from build123d import *

# Parameters (mm, degrees)
SKETCH1_W           = 50
SKETCH1_H           = 5
BOSS_EXTRUDE1_DEPTH = 50
SKETCH2_R           = 8
CUT_EXTRUDE1_DEPTH  = 50
SKETCH3_R           = 5
SKETCH3_R_2         = 4
BOSS_EXTRUDE2_DEPTH = 19
BOSS_EXTRUDE4_DEPTH = 19


with BuildPart() as part:
    # Sketch1 → Boss-Extrude1 (new body)
    with BuildSketch(Plane.XY):
        with Locations((25, -2.5)):
            Rectangle(SKETCH1_W, SKETCH1_H)
    extrude(amount=-BOSS_EXTRUDE1_DEPTH)

    # Sketch2 → Cut-Extrude1 (cut)
    with BuildSketch(Plane.XY):
        Circle(SKETCH2_R)
    extrude(amount=-CUT_EXTRUDE1_DEPTH, mode=Mode.SUBTRACT)



with BuildPart() as body_2:
    # Sketch3 → Boss-Extrude2 (new body)
    with BuildSketch(Plane(origin=(0, 0, -15.5), x_dir=(-1, 0, 0), z_dir=(0, 0, -1))):
        Circle(SKETCH3_R)
        Circle(SKETCH3_R_2, mode=Mode.SUBTRACT)
    extrude(amount=BOSS_EXTRUDE2_DEPTH)


with BuildPart() as part_1:
    add(part.part)

    add(body_2.part)  # Boss-Extrude4 merges body 2
    # Sketch8 → Boss-Extrude4 (add)
    with BuildSketch(Plane(origin=(0, 0, -34.5), x_dir=(-1, 0, 0), z_dir=(0, 0, -1))):
        with BuildLine():
            Line((-4, 0), (-10, 0))
            Line((-10, 0), (-10, -5))
            Line((-10, -5), (0, -5))
            Line((0, -5), (0, -4))
            ThreePointArc((0, -4), (-2.828427125, -2.828427125), (-4, 0))
        make_face()
    extrude(amount=-BOSS_EXTRUDE4_DEPTH)


solid = part_1.part
Work out the finished part from the listing and answer in its coordinate system (mm). A direction names the side the tool comes from. Round coordinates to 2 decimals unless told otherwise and drop trailing zeros. Loops run counter-clockwise (first coordinate to the right, second up) from the corner with the lowest first, then second, coordinate; pieces in that order, holes last. Notation, with made-up numbers: (55.5, 8) -> (77.5, 8) arc R27 cw to (77.5, 28) -> close; hole circle Ø6 at (21.5, 62.25). An arc over 180 degrees is marked (long way). Use one line per item in the form item = value.
(1) Find section D-D on y = -2.5. Give the vertices of the cut face in (x, z).
Answer list:
outline = (-4.33, -34.5) -> (-3.12, -34.5) -> (-3.12, -15.5) -> (-4.33, -15.5) -> close; (3.12, -34.5) -> (7.6, -34.5) -> (7.6, -50) -> (50, -50) -> (50, 0) -> (7.6, 0) -> (7.6, -15.5) -> (3.12, -15.5) -> close
(2) Find section B-B on y = 3.25. Give the vertices of the cut face in (x, z).
Answer list:
outline = (-3.8, -34.5) -> (-2.33, -34.5) -> (-2.33, -15.5) -> (-3.8, -15.5) -> close; (2.33, -34.5) -> (3.8, -34.5) -> (3.8, -15.5) -> (2.33, -15.5) -> close
(3) A tool of negligible diameter and unlimited length cuts with its end or side. For faces 4 (the cylindrical face through (-4, 3, -25)), 5 (the flat face through (4, -2, -34.5)), 6 (the cylindrical face through (7.536, -2.685, -7.642)), from which of +Z, -Z, +X, -X, +Y, -Y can it reach the whole face along a straight path? Write none if from no direction.
Answer list:
face_4 = +Z, -Z
face_5 = -Z, -X, +Y
face_6 = +Z, -X, +Y
(4) For a pull along X with two mould halves and no side action, classify faces 1 (the cylindrical face through (7.536, -2.685, -42.142)), 2 (the flat face through (50, -3, -25)), 3 (the flat face through (27, 0, -25)) as released by +X, released by -X, zero draft, split by the parting line, or undercut.
Answer list:
face_1 = released by -X
face_2 = released by +X
face_3 = zero draft
(5) A flat-ended cylindrical pin translates along its axis: P1, Ø2, axis at y = -3, z = -32.5, coming from the -X side. Find the tip coordinate at first contact, or state that the pin passes through.
Answer list:
P1 = -4.58
(6) Find section A-A on z = -32. Give the vertices of the cut face in (x, y), then the cut area to 3 significant figures.
Answer list:
outline = (0, -5) -> (50, -5) -> (50, 0) -> (5, 0) arc R5 ccw (long way) to start; hole circle Ø8 at (0, 0)
area = 259 mm2
(7) Find section C-C on x = 45. Give the vertices of the cut face in (y, z), then the cut area to 3 significant figures.
Answer list:
outline = (-5, -50) -> (0, -50) -> (0, 0) -> (-5, 0) -> close
area = 250 mm2
(8) Straight lines are drawn through the part: line 1 (Y direction, x = 0, z = -27); line 2 (Y direction, x = 15.5, z = -42); line 3 (Z direction, x = 6, y = -3). For each, find the intervals that lie inside material, in ascending order.
Answer list:
line_1 = -5 to -4, 4 to 5
line_2 = -5 to 0
line_3 = -34.5 to -15.5
